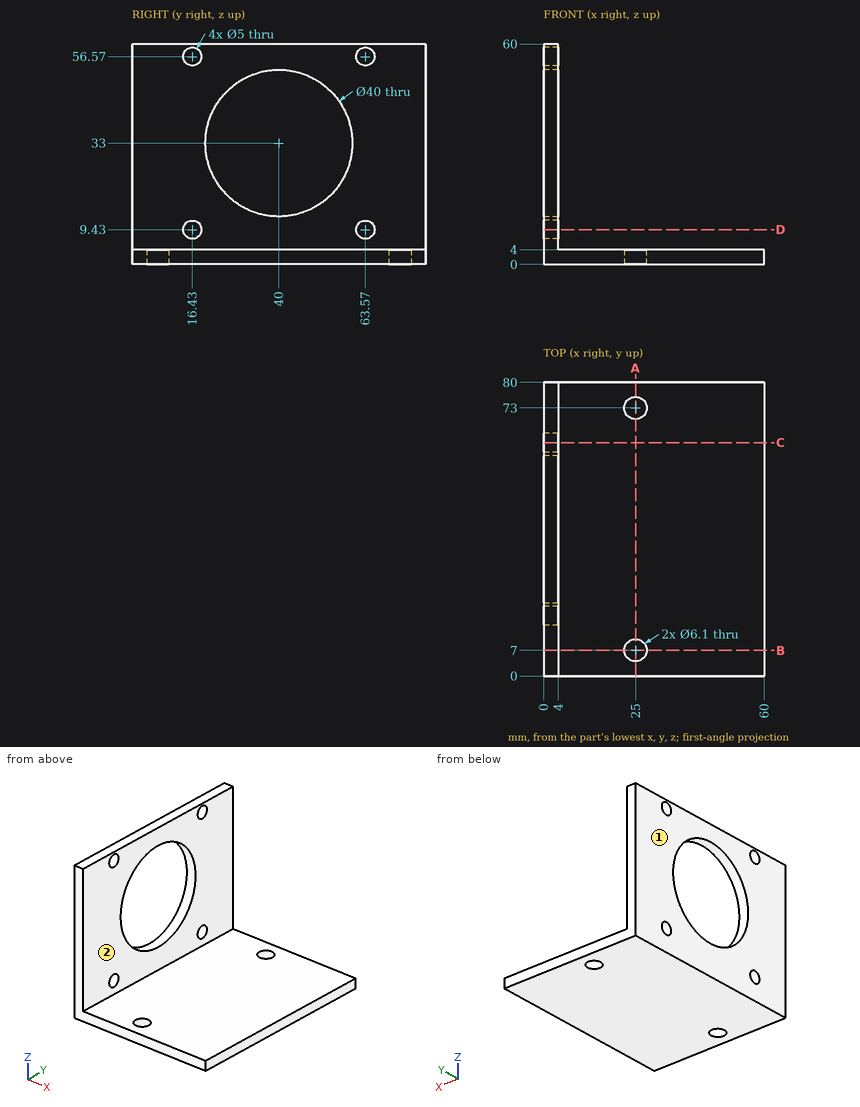
Job drawing, mm, ordinate dimensions from the low corner. One solid piece. A direction names the side the tool comes from. Coordinates: 2 decimals unless noted, no trailing zeros. Write each loop counter-clockwise with the first axis right and the second up, starting at its lowest first coordinate (ties: lowest second). Pieces come first, ordered by that corner, then holes.
Item 1: Pin check, flat tips, straight feed: pin 1 (3 mm diameter, centred on y = 63.57, z = 9.43, fed in from -X); pin 2 (6.5 mm diameter, centred on y = 16.43, z = 9.43, fed in from +X). Stop position of each tip, or through.
Item 2: Slice it at D-D (z = 9.43). Write the cut outline in (x, y), and give its area (3 significant figures).
Item 3: Slice it at C-C (y = 63.57). Write the cut outline in (x, z), and give its area (3 significant figures).
Item 4: Probe line 1 (Z direction, x = 1.15, y = 63.57); line 2 (Y direction, x = 25, z = 3.25); line 3 (X direction, y = 76.5, z = 9). List the from-to ranges inside material, lowest first.
Item 5: Slice it at B-B (y = 7). Write the cut outline in (x, z).
Item 6: Which spindle directions (+Z, -Z, +X, -X, +Y, -Y) get a long thin tool onto all of the face, cutting with end or side? Do the marked faces 1 and 2. Say none if no direction does.
Item 7: Slice it at A-A (x = 25). Write the cut outline in (y, z), and give its area (3 significant figures).
Results found:
1. pin 1: passes through
1. pin 2: stops at x = 4
2. outline: (0, 0) - (4, 0) - (4, 13.93) - (0, 13.93) - close; (0, 18.93) - (4, 18.93) - (4, 61.07) - (0, 61.07) - close; (0, 66.07) - (4, 66.07) - (4, 80) - (0, 80) - close
2. area: 280 mm2
3. outline: (0, 0) - (60, 0) - (60, 4) - (4, 4) - (4, 6.93) - (0, 6.93) - close; (0, 11.93) - (4, 11.93) - (4, 54.07) - (0, 54.07) - close; (0, 59.07) - (4, 59.07) - (4, 60) - (0, 60) - close
3. area: 424 mm2
4. line 1: z = 0 to 6.93, 11.93 to 54.07, 59.07 to 60
4. line 2: y = 0 to 3.95, 10.05 to 69.95, 76.05 to 80
4. line 3: x = 0 to 4
5. outline: (0, 0) - (21.95, 0) - (21.95, 4) - (4, 4) - (4, 60) - (0, 60) - close; (28.05, 0) - (60, 0) - (60, 4) - (28.05, 4) - close
6. face 1: +Z, -Z, -X, +Y, -Y
6. face 2: +Z, +X, +Y, -Y
7. outline: (0, 0) - (3.95, 0) - (3.95, 4) - (0, 4) - close; (10.05, 0) - (69.95, 0) - (69.95, 4) - (10.05, 4) - close; (76.05, 0) - (80, 0) - (80, 4) - (76.05, 4) - close
7. area: 271 mm2
